The figure shows three views and two pictorial views of one solid part (mm, origin at its lowest corner). Answer the questions. A direction names the side the tool comes from. Round coordinates to 2 decimals unless told otherwise and drop trailing zeros. Write each loop counter-clockwise with the first axis right and the second up, starting at its lowest first coordinate (ties: lowest second). Pieces come first, ordered by that corner, then holes.
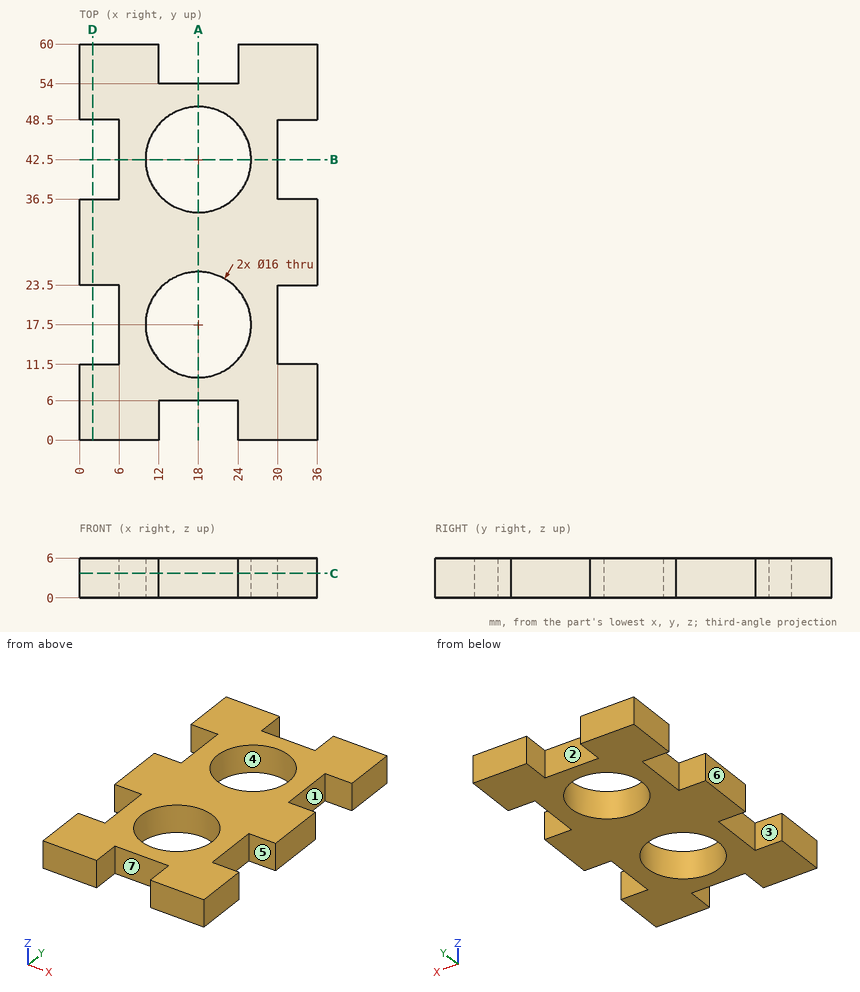
Q1. Straight lines are drawn through the part: probe 1 along Y at (x, z) = (4, 0.95); probe 2 along Y at (x, z) = (18, 1.4); probe 3 along X at (y, z) = (23, 4.95). For each, find the intervals that lie inside material, in ascending order.
Verdict:
probe 1: y = 0 to 11.5, 23.5 to 36.5, 48.5 to 60
probe 2: y = 6 to 9.5, 25.5 to 34.5, 50.5 to 54
probe 3: x = 6 to 12.19, 23.81 to 30
Q2. Section D-D (x = 2) is taken. Determine the outline of the cut face in (y, z).
Verdict:
outline: (0, 0) - (11.5, 0) - (11.5, 6) - (0, 6) - close; (23.5, 0) - (36.5, 0) - (36.5, 6) - (23.5, 6) - close; (48.5, 0) - (60, 0) - (60, 6) - (48.5, 6) - close
Q3. Section C-C (z = 3.7) is taken. State how many separate pieces and enclosed holes the cut face has, then the cut area to 3 significant figures.
Verdict:
separate pieces: 1
enclosed holes: 2
area: 1,330 mm2
Q4. Section A-A (x = 18) is taken. Determine the outline of the cut face in (y, z).
Verdict:
outline: (6, 0) - (9.5, 0) - (9.5, 6) - (6, 6) - close; (25.5, 0) - (34.5, 0) - (34.5, 6) - (25.5, 6) - close; (50.5, 0) - (54, 0) - (54, 6) - (50.5, 6) - close
Q5. Flat-ended cylindrical pins translate along their axes: pin 1 Ø1.8 at (x, z) = (19, 3.5) entering from -Y; pin 2 Ø3 at (y, z) = (16, 4.5) entering from +X. Find the tip coordinate at first contact, or state that the pin passes through.
Verdict:
pin 1: stops at y = 6
pin 2: stops at x = 30
Q6. Which of the six approach directions +Z, -Z, +X, -X, +Y, -Y give full straight-line access (tool end or side, diameter ignored) to the marked faces 1, 2, 3 and 4?
Verdict:
face 1: +Z, -Z, +X
face 2: +Z, -Z, +Y
face 3: +Z, -Z, -X
face 4: +Z, -Z
Q7. Determine the mould class of the marked faces 5, 6 and 7 for opening direction Y: pulls with the +Y half, pulls with the -Y half, needs draft (parallel to the pull), parting line crosses it, or undercut.
Verdict:
face 5: undercut
face 6: needs draft
face 7: pulls with the -Y half
Q8. Section B-B (y = 42.5) is taken. Determine the outline of the cut face in (x, z).
Verdict:
outline: (6, 0) - (10, 0) - (10, 6) - (6, 6) - close; (26, 0) - (30, 0) - (30, 6) - (26, 6) - close
